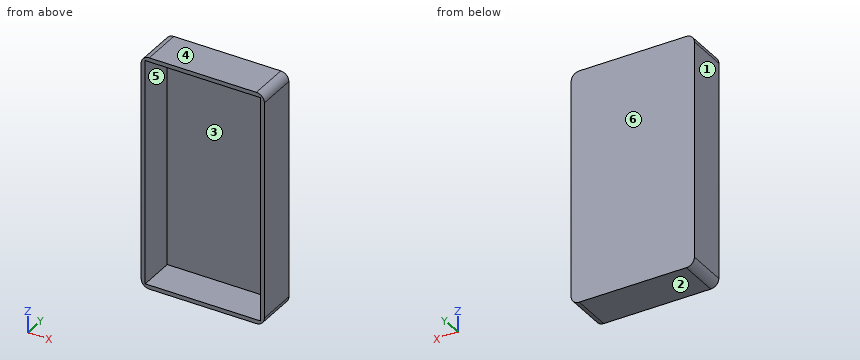
```python
from build123d import *

# Parameters (mm, degrees)
F0_W     = 77.455164
F0_H     = 146.724008
F1_DEPTH = 12.7
F2_T     = -2.54
F3_R     = 5.08


with BuildPart() as f1:
    # F0 (on Front) → F1 (new body, symmetric)
    with BuildSketch(Plane.XZ):
        Rectangle(F0_W, F0_H)
    extrude(amount=F1_DEPTH, both=True)

    # F2
    f2_openings = [f1.faces().sort_by_distance(p)[0] for p in [
        (0, -12.7, 0),
    ]]
    offset(amount=F2_T, openings=f2_openings)

    # F3
    f3_edges = [f1.edges().sort_by_distance(p)[0] for p in [
        (38.727582, 0, 73.362004),
        (38.727582, 0, -73.362004),
        (-38.727582, 0, 73.362004),
        (-38.727582, 0, -73.362004),
    ]]
    fillet(f3_edges, radius=F3_R)


solid = f1.part
```
Here's how the part is built. I have some questions about the finished solid (model axes, mm). Face numbers are marked on the shaded views. A direction names the side the tool comes from. Give positions to 0.01 mm unless a question says otherwise; leave off trailing zeros. Write each loop counter-clockwise with the first axis right and the second up, starting at its lowest first coordinate (ties: lowest second). Pieces come first, ordered by that corner, then holes.
(1) Imagine slicing it at B-B, the plane x = -5.5. Write out the boundary of the cut face in (y, z), and give its area (3 significant figures).
Output values:
outline: (-12.7, -73.36) - (12.7, -73.36) - (12.7, 73.36) - (-12.7, 73.36) - (-12.7, 70.82) - (10.16, 70.82) - (10.16, -70.82) - (-12.7, -70.82) - close
area: 489 mm2
(2) Imagine slicing it at C-C, the plane z = -43. Write out the boundary of the cut face in (x, y), and give its area (3 significant figures).
Output values:
outline: (-38.73, -12.7) - (-36.19, -12.7) - (-36.19, 10.16) - (36.19, 10.16) - (36.19, -12.7) - (38.73, -12.7) - (38.73, 12.7) - (-38.73, 12.7) - close
area: 313 mm2
(3) If I drill on L1, parallel to X at y = 10, z = 54.5; L2, parallel to Z at x = 27, y = 3.75; L3, parallel to Y at x = 24.5, z = -17.5, over which ranges is the centre line in solid material (lowest first)?
Output values:
L1: x = -38.73 to -36.19, 36.19 to 38.73
L2: z = -73.36 to -70.82, 70.82 to 73.36
L3: y = 10.16 to 12.7
(4) On a 3-axis mill with a long thin cutter (end or side, diameter ignored), from which of +Z, -Z, +X, -X, +Y, -Y can I reach the whole of each face in a straight line? I mean the marked faces 5 and 6. Say none if no direction works.
Output values:
face 5: -Y
face 6: +Z, -Z, +X, -X, +Y
(5) Imagine slicing it at A-A, the plane y = -1.75. Write out the boundary of the cut face in (x, z), and give its area (3 significant figures).
Output values:
outline: (-38.73, -68.28) arc R5.08 ccw to (-33.65, -73.36) - (33.65, -73.36) arc R5.08 ccw to (38.73, -68.28) - (38.73, 68.28) arc R5.08 ccw to (33.65, 73.36) - (-33.65, 73.36) arc R5.08 ccw to (-38.73, 68.28) - close; hole (-36.19, -70.82) - (36.19, -70.82) - (36.19, 70.82) - (-36.19, 70.82) - close
area: 1,090 mm2
(6) Will this pin go through, and if not, where does the flat tip stop? pin 1 (1.5 mm diameter, centred on x = -13.5, z = -11.5, fed in from -Y).
Output values:
pin 1: stops at y = 10.16
(7) Thinking about a two-plate mould opening in Z: for the marked faces 1, 2, 3 and 4, which applies, pulls with the +Z half, pulls with the -Z half, needs draft (parallel to the pull), parting line crosses it, or undercut?
Output values:
face 1: needs draft
face 2: pulls with the -Z half
face 3: undercut
face 4: pulls with the +Z half
